For this review, take the finished solid that the model builds, in its own axes (mm). Face numbers are marked on the shaded views. A direction names the side the tool comes from. Coordinates: 2 decimals unless noted, no trailing zeros. Order: outer loops, then holes, each group sorted by start corner. A loop starts at its lowest first (then second) coordinate and runs counter-clockwise, first axis right, second up. Notation, with made-up numbers: M 3,7.5 L 19,7.5 A21 ccw 19,12.5 Z; hole C -33.5,-26.5 d3. An arc over 180 degrees is marked long. Use CSV: the item, a comma, the result in double quotes.
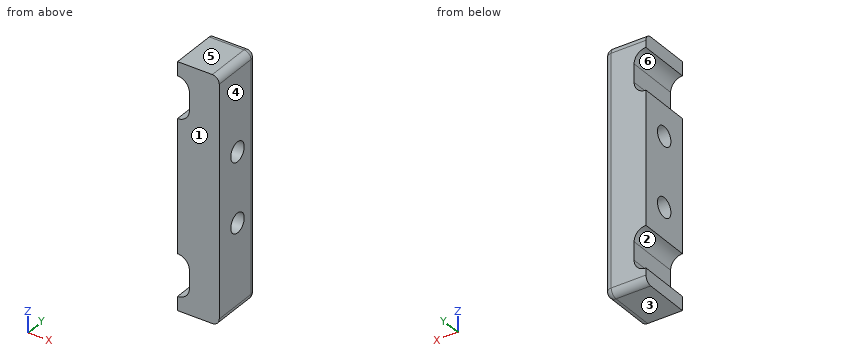
```python
from build123d import *

# Parameters (mm, degrees)
BASE_DEPTH           = 7.6
SKETCH2_R            = 1.4
SCREW_HOLES_DEPTH    = 21.000249998
F_1MM_EDGE_FILLETS_R = 1


with BuildPart() as part:
    # Sketch1 → Base (new body)
    with BuildSketch(Plane(origin=(0, 0, 0), x_dir=(1, 0, 0), z_dir=(0, 1, 0))):
        with BuildLine():
            Line((-6, 17.5), (-6, 15.5))
            ThreePointArc((-6, 15.5), (-4.797918472, 15.002081528), (-4.3, 13.8))
            Line((-4.3, 13.8), (-4.3, 11.2))
            ThreePointArc((-4.3, 11.2), (-4.797918472, 9.997918472), (-6, 9.5))
            Line((-6, 9.5), (-6, -9.5))
            ThreePointArc((-6, -9.5), (-4.797918472, -9.997918472), (-4.3, -11.2))
            Line((-4.3, -11.2), (-4.3, -13.8))
            ThreePointArc((-4.3, -13.8), (-4.797918472, -15.002081528), (-6, -15.5))
            Line((-6, -15.5), (-6, -17.5))
            Line((-6, -17.5), (0, -17.5))
            Line((0, -17.5), (0, 17.5))
            Line((0, 17.5), (-6, 17.5))
        make_face()
    extrude(amount=BASE_DEPTH)

    # Sketch2 → Screw Holes (cut, through all)
    with BuildSketch(Plane.ZY.offset(6)):
        with Locations((-5, 3.8)):
            Circle(SKETCH2_R)
        with Locations(Location((5, 3.8, 0), (0, 0, 180))):
            Circle(SKETCH2_R)
    extrude(amount=-SCREW_HOLES_DEPTH, mode=Mode.SUBTRACT)

    # 1mm Edge Fillets
    f_1mm_edge_fillets_edges = [part.edges().sort_by_distance(p)[0] for p in [
        (0, 3.8, -17.5),
        (0, 3.8, 17.5),
        (-3, 7.6, 17.5),
        (0, 7.6, 0),
        (-3, 7.6, -17.5),
    ]]
    fillet(f_1mm_edge_fillets_edges, radius=F_1MM_EDGE_FILLETS_R)


solid = part.part
```
Item 1: Add section C-C on z = -6. State the section outline as (x, y) points.
Solutions:
outline,"M -6,0 L 0,0 L 0,2.82 L -6,2.82 Z; M -6,4.78 L 0,4.78 L 0,6.6 A1 ccw -1,7.6 L -6,7.6 Z"
Item 2: Add section D-D on x = -2.35. State the section outline as (y, z) points, and give its area (3 significant figures).
Solutions:
outline,"M 0,-17.5 L 6.6,-17.5 A1 ccw 7.6,-16.5 L 7.6,16.5 A1 ccw 6.6,17.5 L 0,17.5 Z; hole C 3.8,-5 d2.8; hole C 3.8,5 d2.8"
area,"253 mm^2"
Item 3: Add section B-B on y = 3.8. State the section outline as (x, z) points.
Solutions:
outline,"M -6,-17.5 L -1,-17.5 A1 ccw 0,-16.5 L 0,-6.4 L -6,-6.4 L -6,-9.5 A1.7 cw -4.3,-11.2 L -4.3,-13.8 A1.7 cw -6,-15.5 Z; M -6,-3.6 L 0,-3.6 L 0,3.6 L -6,3.6 Z; M -6,6.4 L 0,6.4 L 0,16.5 A1 ccw -1,17.5 L -6,17.5 L -6,15.5 A1.7 cw -4.3,13.8 L -4.3,11.2 A1.7 cw -6,9.5 Z"
Item 4: Add section A-A on x = -5.2. State the section outline as (y, z) points.
Solutions:
outline,"M 0,-17.5 L 6.6,-17.5 A1 ccw 7.6,-16.5 L 7.6,-15.3 L 0,-15.3 Z; M 0,-9.7 L 7.6,-9.7 L 7.6,9.7 L 0,9.7 Z; M 0,15.3 L 7.6,15.3 L 7.6,16.5 A1 ccw 6.6,17.5 L 0,17.5 Z; hole C 3.8,-5 d2.8; hole C 3.8,5 d2.8"
Item 5: Clearance check with flat-ended pins moving along their axes: pin 1 Ø1 at (x, z) = (-5.5, -11.5) entering from -Y; pin 2 Ø2 at (y, z) = (4, 12.5) entering from -X. State where each tip first meets the part, or that it passes through.
Solutions:
pin 1,"through"
pin 2,"x = -4.3"
Item 6: To check wall thickness, follow line 1 along Y through (x, z) = (-3.4, -5); line 2 along Z through (x, y) = (-4.8, 5.75); line 3 along X through (y, z) = (5.25, 13). State the ranges of each line that lie inside material, in increasing order. Write a range as [from, to].
Solutions:
line 1,"[0, 2.4], [5.2, 7.6]"
line 2,"[-17.5, -15], [-10, 10], [15, 17.5]"
line 3,"[-4.3, 0]"
Item 7: Draft analysis for pull direction Z (two halves, no side actions). For the marked faces 3, 4, 5 and 6, state which applies: released by +Z, released by -Z, zero draft, split by the parting line, or undercut.
Solutions:
face 3,"released by -Z"
face 4,"zero draft"
face 5,"released by +Z"
face 6,"undercut"
Item 8: For the marked faces 1 and 2, list the 3-axis set-ups (+Z, -Z, +X, -X, +Y, -Y) from which the entire face can be reached by the end or side of a thin tool; tool diameter is ignored.
Solutions:
face 1,"+Z, -Z, +X, -X, -Y"
face 2,"-X, +Y, -Y"
